Part model, mm, in its own coordinate system. A direction names the side the tool comes from. Coordinates: 2 decimals unless noted, no trailing zeros. Write each loop counter-clockwise with the first axis right and the second up, starting at its lowest first coordinate (ties: lowest second). Pieces come first, ordered by that corner, then holes. Notation, with made-up numbers: (36.25, 1.25) - (80.25, 1.25) arc R16 cw to (80.25, 22.25) - close; hole circle Ø1 at (44, -39). An arc over 180 degrees is marked (long way). Use a Markdown table: item, result.
```python
from build123d import *

# Parameters (mm, degrees)
F0_W     = 50.8
F0_H     = 44.824883
F1_DEPTH = 25.4
F3_D     = 12.7
F4_W     = 32.221506
F4_H     = 28.573785
F5_DEPTH = 12.954
F6_R     = 9.448071
F7_DEPTH = 9.398


with BuildPart() as f1:
    # F0 (on Front) → F1 (new body)
    with BuildSketch(Plane.XZ):
        with Locations((-25.4, 22.412441)):
            Rectangle(F0_W, F0_H)
    extrude(amount=F1_DEPTH)

    # F3 (through all)
    with Locations(Plane.XY.offset(44.824883)):
        with Locations((-25.40575, -11.502657)):
            Hole(F3_D / 2)

    # F4 (on face) → F5 (join)
    with BuildSketch(Plane.XZ.offset(25.4)):
        with Locations((-25.191973, 23.439532)):
            Rectangle(F4_W, F4_H)
    extrude(amount=F5_DEPTH)

    # F6 (on face) → F7 (join)
    with BuildSketch(Plane.YZ):
        with Locations((-12.772681, 23.858404)):
            Circle(F6_R)
    extrude(amount=F7_DEPTH)


solid = f1.part
```
Item 1: Drop flat-ended pins along their axis: P1, Ø4, axis at y = -12, z = 12, coming from the +X side; P2, Ø6, axis at x = 0.5, z = 39, coming from the -Y side; P3, Ø4, axis at y = -30.5, z = 23.5, coming from the -X side; P4, Ø20.5, axis at x = -25.41, y = -11.5, coming from the -Z side. Give the stop position or say it passes through.
From the geometry:
| item | result |
|---|---|
| P1 | x = 0 |
| P2 | y = -25.4 |
| P3 | x = -41.3 |
| P4 | z = 0 |
Item 2: Band-saw the part on C-C, the plane x = -39.5. Give the cut face in (y, z).
From the geometry:
| item | result |
|---|---|
| outline | (-38.35, 9.15) - (-25.4, 9.15) - (-25.4, 0) - (0, 0) - (0, 44.82) - (-25.4, 44.82) - (-25.4, 37.73) - (-38.35, 37.73) - close |
Item 3: Two-plate mould, pull along Y, no slides. Class faces 4 (the face through (-20.37, -15.37, 22.1)), 5 (the face through (4.63, -19.74, 30.24)), 6 (the face through (0, -13, 12)): pulls with the +Y half, pulls with the -Y half, needs draft (parallel to the pull), parting line crosses it, or undercut.
From the geometry:
| item | result |
|---|---|
| face 4 | undercut |
| face 5 | parting line crosses it |
| face 6 | needs draft |
Item 4: Drill centre lines: probe 1 along X at (y, z) = (-5, 38.5); probe 2 along X at (y, z) = (-26.5, 11); probe 3 along Y at (x, z) = (-30.5, 12). Where is each one in solid material? Low to high.
From the geometry:
| item | result |
|---|---|
| probe 1 | -50.8 to 0 |
| probe 2 | -41.3 to -9.08 |
| probe 3 | -38.35 to -15.29, -7.71 to 0 |
Item 5: Band-saw the part on D-D, the plane y = -27. Give the cut face in (x, z).
From the geometry:
| item | result |
|---|---|
| outline | (-41.3, 9.15) - (-9.08, 9.15) - (-9.08, 37.73) - (-41.3, 37.73) - close |
Item 6: Band-saw the part on A-A, the plane z = 35. Give the cut face in (x, y), then the cut area to 3 significant figures.
From the geometry:
| item | result |
|---|---|
| outline | (-50.8, -25.4) - (-41.3, -25.4) - (-41.3, -38.35) - (-9.08, -38.35) - (-9.08, -25.4) - (0, -25.4) - (0, 0) - (-50.8, 0) - close; hole circle Ø12.7 at (-25.41, -11.5) |
| area | 1,580 mm^2 |
Item 7: Which spindle directions (+Z, -Z, +X, -X, +Y, -Y) get a long thin tool onto all of the face, cutting with end or side? Do faces 1 (the face through (-25, -32, 9.153)), 2 (the face through (-41.303, -32, 23)), 3 (the face through (-9.081, -32, 23)). Say none if no direction does.
From the geometry:
| item | result |
|---|---|
| face 1 | -Z, +X, -X, -Y |
| face 2 | +Z, -Z, -X, -Y |
| face 3 | +Z, -Z, +X, -Y |
Item 8: Band-saw the part on B-B, the plane x = -24. Give the cut face in (y, z).
From the geometry:
| item | result |
|---|---|
| outline | (-38.35, 9.15) - (-25.4, 9.15) - (-25.4, 0) - (-17.7, 0) - (-17.7, 44.82) - (-25.4, 44.82) - (-25.4, 37.73) - (-38.35, 37.73) - close; (-5.31, 0) - (0, 0) - (0, 44.82) - (-5.31, 44.82) - close |
